```python
from build123d import *

# Parameters (mm, degrees)
BOSS_EXTRUDE1_DEPTH = 2
BOSS_EXTRUDE2_DEPTH = 0.0001


with BuildPart() as part:
    # Sketch1 → Boss-Extrude1 (new body)
    with BuildSketch(Plane.XY):
        Polygon((-38, -35), (-26.452994616, -55), (26.452994616, -55), (38, -35), (38, 35), (-38, 35), align=None)
    extrude(amount=BOSS_EXTRUDE1_DEPTH)

    # Sketch2 → Boss-Extrude2 (add)
    with BuildSketch(Plane.XY.offset(2)):
        Polygon((-38, 7.945483094), (-10.149076909, 35), (5.637899584, 35), (-38, -7.390059683), align=None)
        Polygon((-38, -35.272864732), (34.341493208, 35), (38, 35), (38, 23.218347826), (-32.226497308, -45), align=None)
        Polygon((-13.81727456, -55), (38, -4.664457223), (38, -20), (1.969701933, -55), align=None)
    extrude(amount=BOSS_EXTRUDE2_DEPTH)


solid = part.part
```
Build history of the part. All positions in model axes, mm. A direction names the side the tool comes from. Coordinates: 2 decimals unless noted, no trailing zeros. Order: outer loops, then holes, each group sorted by start corner. A loop starts at its lowest first (then second) coordinate and runs counter-clockwise, first axis right, second up.
Item 1: Tool access for faces 1 (the flat face through (24, -44, 2)), 2 (the flat face through (-32.307, -44.86, 0.986)): list every direction of +Z, -Z, +X, -X, +Y, -Y with a clear straight run to the whole face (end or side of a thin tool).
Filled in:
face 1: +Z, +X, -X, +Y, -Y
face 2: -Z, -X, -Y
Item 2: Drill centre lines: L1, parallel to X at y = -48, z = 0.3; L2, parallel to Y at x = -31.5, z = 0.55; L3, parallel to X at y = -41, z = 0.45. Where is each one in solid material? Low to high.
Filled in:
L1: x = -30.49 to 30.49
L2: y = -46.26 to 35
L3: x = -34.54 to 34.54
Item 3: Saw through at A-A on z = 1.05. List the corners of the cut face in (x, y), then the cut area to 3 significant figures.
Filled in:
outline: (-38, -35) - (-26.45, -55) - (26.45, -55) - (38, -35) - (38, 35) - (-38, 35) - close
area: 6,610 mm2
